Work out the finished part from the listing and answer in its coordinate system (mm). A direction names the side the tool comes from. Round coordinates to 2 decimals unless told otherwise and drop trailing zeros. Write each loop counter-clockwise with the first axis right and the second up, starting at its lowest first coordinate (ties: lowest second). Pieces come first, ordered by that corner, then holes. Notation, with made-up numbers: M 38,-5 L 85,-5 A15 cw 85,2 Z; hole C 16,-17 d9. An arc over 180 degrees is marked long. Answer in a Markdown table with one row per item.
```python
from build123d import *

# Parameters (mm, degrees)
SKETCH1_W           = 95.25
SKETCH1_H           = 25.4
SKETCH1_W_2         = 69.85
SKETCH1_H_2         = 12.7
BOSS_EXTRUDE1_DEPTH = 15
SKETCH2_W           = 9.525
SKETCH2_H           = 6.35
BOSS_EXTRUDE2_DEPTH = 55
CHAMFER1_SIZE       = 2.54
SKETCH4_W           = 9.525
SKETCH4_H           = 6.35
CUT_EXTRUDE2_DEPTH  = 113.883667995


with BuildPart() as part:
    # Sketch1 → Boss-Extrude1 (new body)
    with BuildSketch(Plane.XY):
        with Locations((-47.625, 12.7)):
            Rectangle(SKETCH1_W, SKETCH1_H)
        with Locations((-47.625, 12.7)):
            Rectangle(SKETCH1_W_2, SKETCH1_H_2, mode=Mode.SUBTRACT)
    extrude(amount=BOSS_EXTRUDE1_DEPTH)

    # Sketch2 → Boss-Extrude2 (add)
    with BuildSketch(Plane.XY.offset(15)):
        with Locations((-90.4875, 9.525)):
            Rectangle(SKETCH2_W, SKETCH2_H)
    extrude(amount=BOSS_EXTRUDE2_DEPTH)

    # Chamfer1
    chamfer1_edges = [part.edges().sort_by_distance(p)[0] for p in [
        (-95.25, 25.4, 7.5),
        (0, 25.4, 7.5),
        (0, 0, 7.5),
        (-95.25, 0, 7.5),
    ]]
    chamfer(chamfer1_edges, length=CHAMFER1_SIZE)

    # Sketch4 → Cut-Extrude2 (cut, through all)
    with BuildSketch(Plane.XY.offset(15)):
        with Locations((-90.4875, 3.175)):
            Rectangle(SKETCH4_W, SKETCH4_H)
    extrude(amount=-CUT_EXTRUDE2_DEPTH, mode=Mode.SUBTRACT)


solid = part.part
```
1. Determine the mould class of faces 1 (the flat face through (-45, 0, 7)), 2 (the flat face through (0, 13, 7)), 3 (the flat face through (-82.55, 13, 7)) for opening direction X: released by +X, released by -X, zero draft, split by the parting line, or undercut.
Calculated:
| item | result |
|---|---|
| face 1 | zero draft |
| face 2 | released by +X |
| face 3 | undercut |
2. Given pin 1 (12.5 mm diameter, centred on x = -38, y = 11.5, fed in from +Z); pin 2 (7.5 mm diameter, centred on x = -89.5, z = 43, fed in from +Y); pin 3 (10 mm diameter, centred on y = 17.5, z = 26.5, fed in from +X) (3 decimals); pin 4 (6 mm diameter, centred on x = -15.5, z = 17, fed in from -Y), each flat-ended and moving along its own axis, determine where each tip first touches the part or whether it passes through.
Calculated:
| item | result |
|---|---|
| pin 1 | stops at z = 15 |
| pin 2 | stops at y = 12.7 |
| pin 3 | stops at x = -85.725 |
| pin 4 | stops at y = 0 |
3. Consider line 1 along Z through (x, y) = (-29, 21.75); line 2 along X through (y, z) = (12.25, 44) (3 decimals); line 3 along Y through (x, z) = (-59, 11). Determine where each line is inside the solid, lowest interval first. Write a range as from..to.
Calculated:
| item | result |
|---|---|
| line 1 | z = 0..15 |
| line 2 | x = -95.25..-85.725 |
| line 3 | y = 0..6.35, 19.05..25.4 |
4. The part is cut by section B-B (x = -24). Determine the outline of the cut face in (y, z), plus the area to 4 significant figures.
Calculated:
| item | result |
|---|---|
| outline | M 0,0 L 6.35,0 L 6.35,15 L 0,15 Z; M 19.05,0 L 25.4,0 L 25.4,15 L 19.05,15 Z |
| area | 190.5 mm² |
5. The part is cut by section A-A (y = 17.5). Determine the outline of the cut face in (x, z).
Calculated:
| item | result |
|---|---|
| outline | M -95.25,0 L -82.55,0 L -82.55,15 L -95.25,15 Z; M -12.7,0 L 0,0 L 0,15 L -12.7,15 Z |
6. The part is cut by section D-D (z = 39). Determine the outline of the cut face in (x, y) (3 decimals).
Calculated:
| item | result |
|---|---|
| outline | M -95.25,6.35 L -85.725,6.35 L -85.725,12.7 L -95.25,12.7 Z |
7. A tool of negligible diameter and unlimited length cuts with its end or side. For faces 4 (the flat face through (-85.725, 9, 42)), 5 (the flat face through (-85.725, 3, 8)), 6 (the flat face through (-91, 12.7, 42)), 7 (the flat face through (-48, 19.05, 7)), from which of +Z, -Z, +X, -X, +Y, -Y can it reach the whole face along a straight path? Write none if from no direction.
Calculated:
| item | result |
|---|---|
| face 4 | +Z, +X, +Y, -Y |
| face 5 | +Z, -Z, -X, -Y |
| face 6 | +Z, +X, -X, +Y |
| face 7 | +Z, -Z |
8. The part is cut by section C-C (y = 7.75). Determine the outline of the cut face in (x, z) (3 decimals).
Calculated:
| item | result |
|---|---|
| outline | M -95.25,0 L -82.55,0 L -82.55,15 L -85.725,15 L -85.725,70 L -95.25,70 Z; M -12.7,0 L 0,0 L 0,15 L -12.7,15 Z |
